Input: part model. Units: mm. Frame: model coordinates. A direction names the side the tool comes from. Coordinates: 2 decimals unless noted, no trailing zeros. Order: outer loops, then holes, each group sorted by start corner. A loop starts at its lowest first (then second) coordinate and runs counter-clockwise, first axis right, second up. Notation, with made-up numbers: (65.5, 51.25) -> (80.5, 51.25) arc R35 ccw to (80.5, 85.25) -> close; hole circle Ø3 at (4.25, 37). An arc over 180 degrees is marked (long way). Use CSV: the item, a comma, the result in double quotes. Start each with the question number.
```python
from build123d import *

# Parameters (mm, degrees)
F8_R      = 1.25
F9_DEPTH  = 36.001
F10_R     = 4.75
F10_R_2   = 1.25
F11_DEPTH = 6
F13_R     = 2.9
F14_DEPTH = 4


with BuildPart() as f2:
    # F0 (on Top) → F2 (revolve)
    with BuildSketch(Plane.XY):
        with BuildLine():
            Line((0, -18), (0, 18))
            ThreePointArc((0, 18), (-18, 0), (0, -18))
        make_face()
    revolve(axis=Axis((0, -0.836778, 0), (0, -1, 0)))

    # F8 (on offset) → F9 (cut, through all)
    with BuildSketch(Plane.XY.offset(18)):
        with Locations((2.5, 0)):
            Circle(F8_R)
    extrude(amount=-F9_DEPTH, mode=Mode.SUBTRACT)

    # F10 (on offset) → F11 (cut)
    with BuildSketch(Plane.XY.offset(-18)):
        Circle(F10_R)
        with Locations((2.5, 0)):
            Circle(F10_R_2, mode=Mode.SUBTRACT)
    extrude(amount=F11_DEPTH, mode=Mode.SUBTRACT)

    # F13 (on offset) → F14 (cut)
    with BuildSketch(Plane.XY.offset(18)):
        with Locations((2.5, 0)):
            Circle(F13_R)
    extrude(amount=-F14_DEPTH, mode=Mode.SUBTRACT)


solid = f2.part
```
1. Section C-C on z = 12. Return loops of the section in (x, y), then the cut area to 3 significant figures.
2. Section A-A on y = 0. Return loops of the section in (x, z).
3. Section D-D on y = 12.5. Return loops of the section in (x, z).
4. Material intervals for line 1 along Y through (x, z) = (0, -13.9); line 2 along Y through (x, z) = (2.5, -6.5); line 3 along X through (y, z) = (0, -14), sorted ascending.
5. Contact query for flat-ended pins moving along their axis: P1, Ø5, axis at x = 2.5, y = 0, coming from the +Z side; P2, Ø5, axis at x = -8.5, z = -3, coming from the +Y side; P3, Ø8, axis at y = 2, z = -14, coming from the +X side. Output: stop coordinate, or through.
6. Section B-B on x = 2. Return loops of the section in (y, z).
7. Access query for faces 1 (the face through (0, 0, -12)), 2 (the face through (3.69, 0.38, 1.18)), 3 (the face through (-0.4, 0.1, 16)). Directions: +Z, -Z, +X, -X, +Y, -Y. A direction counts if a zero-diameter tool reaches every point of the face in a straight line with its end or side. Return the directions, or none.
Values follow:
1,outline,"circle Ø26.83 at (0, 0); hole circle Ø2.5 at (2.5, 0)"
1,area,"561 mm2"
2,outline,"(-4.75, -17.36) -> (-4.75, -12) -> (1.25, -12) -> (1.25, 14) -> (-0.4, 14) -> (-0.4, 18) arc R18 ccw to start; (3.75, -12) -> (4.75, -12) -> (4.75, -17.36) arc R18 ccw to (5.4, 17.17) -> (5.4, 14) -> (3.75, 14) -> close"
3,outline,"circle Ø25.9 at (0, 0)"
4,line 1,"y = -11.44 to -4.75, 4.75 to 11.44"
4,line 2,"y = -16.6 to -1.25, 1.25 to 16.6"
4,line 3,"x = -11.31 to -4.75, 4.75 to 11.31"
5,P1,"stops at z = 14"
5,P2,"stops at y = 16.78"
5,P3,"stops at x = 14.87"
6,outline,"(-4.31, -17.36) -> (-4.31, -12) -> (-1.15, -12) -> (-1.15, 14) -> (-2.86, 14) -> (-2.86, 17.66) arc R17.89 ccw to start; (1.15, -12) -> (4.31, -12) -> (4.31, -17.36) arc R17.89 ccw to (2.86, 17.66) -> (2.86, 14) -> (1.15, 14) -> close"
7,face 1,"-Z"
7,face 2,"+Z, -Z"
7,face 3,"+Z"
